Here's the drawing with two shaded views (mm, measured from the low corner). I have some questions. A direction names the side the tool comes from. Give positions to 0.01 mm unless a question says otherwise; leave off trailing zeros. Order: outer loops, then holes, each group sorted by start corner. A loop starts at its lowest first (then second) coordinate and runs counter-clockwise, first axis right, second up. Notation, with made-up numbers: (-32.75, 31) - (-7.75, 31) arc R21 cw to (-7.75, 37) - close; hole circle Ø10 at (61, 82.5). An arc over 180 degrees is marked (long way). Use one line per item in the form item = value. Start each with the question number.
1) For pin 1 (6.5 mm diameter, centred on y = 9.5, z = 13.5, fed in from +X); pin 2 (3 mm diameter, centred on x = 6.35, z = 6.35, fed in from -Y); pin 3 (4 mm diameter, centred on x = 22, y = 3.5, fed in from +Z), each with a flat end and sliding along its axis, tell me the tip position at first contact or that it passes through.
2) Suppose I cut it at A-A, the plane x = 6.35. Write out the boundary of the cut face in (y, z), and give its area (3 significant figures).
3) Please list where these lines run through material, in increasing order: probe 1 along Z at (x, y) = (6.35, 6.5); probe 2 along Z at (x, y) = (3.25, 6.35); probe 3 along Z at (x, y) = (6.35, 5).
4) Which directions (+Z, -Z, +X, -X, +Y, -Y) give clear straight access to the entire face, cutting with the end or side of a thin tool? Please do the marked faces 5 and 6.
5) We'd pull the mould along Y, two halves only. Please class the marked faces 1, 2, 3 and 4: released by +Y, released by -Y, zero draft, split by the parting line, or undercut.
6) Suppose I cut it at C-C, the plane z = 6.35. Write out the boundary of the cut face in (x, y), and give its area (3 significant figures).
7) Suppose I cut it at B-B, the plane y = 6.35. Write out the boundary of the cut face in (x, z), and give its area (3 significant figures).
8) Suppose I cut it at D-D, the plane x = 3. Write out the boundary of the cut face in (y, z), and give its area (3 significant figures).
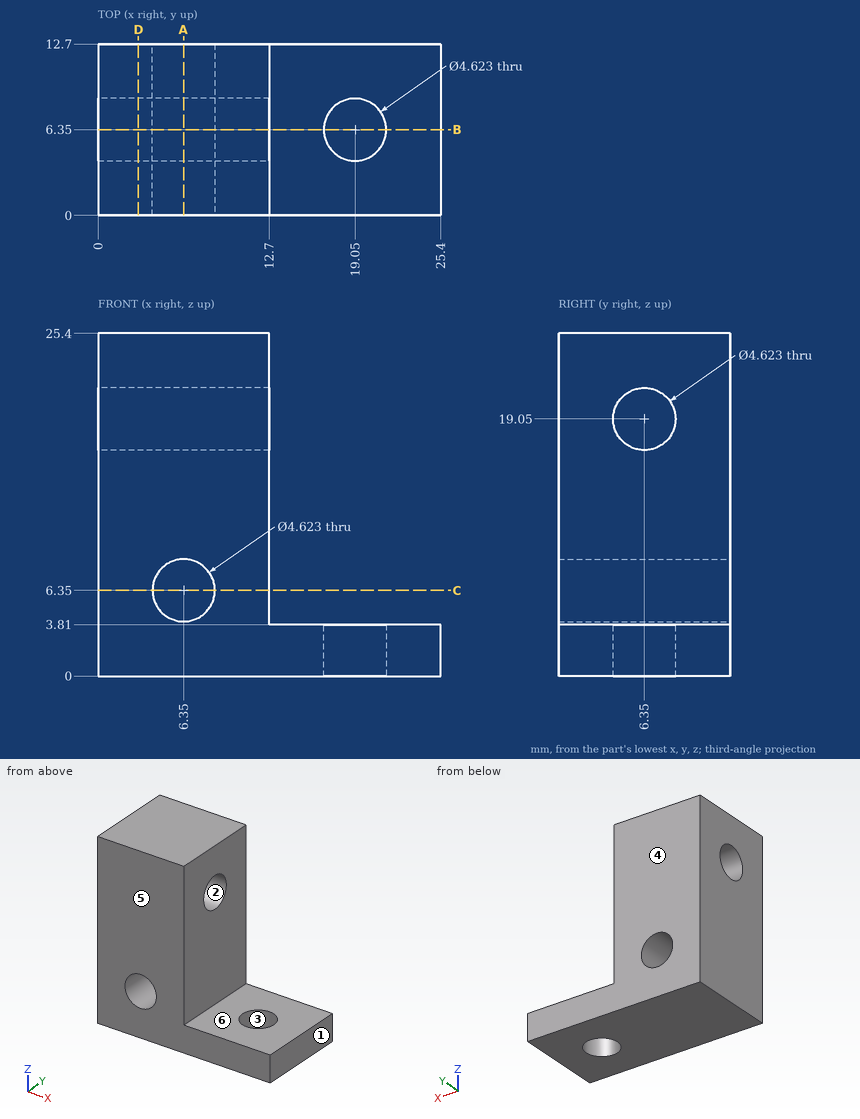
Result sheet:
q1.pin_1 = 12.7
q1.pin_2 = through
q1.pin_3 = 3.81
q2.outline = (0, 0) - (12.7, 0) - (12.7, 4.04) - (0, 4.04) - close; (0, 8.66) - (12.7, 8.66) - (12.7, 25.4) - (0, 25.4) - close; hole circle Ø4.62 at (6.35, 19.05)
q2.area = 247 mm²
q3.probe_1 = 0 to 4.04, 8.66 to 16.74, 21.36 to 25.4
q3.probe_2 = 0 to 16.74, 21.36 to 25.4
q3.probe_3 = 0 to 4.04, 8.66 to 17.17, 20.93 to 25.4
q4.face_5 = +Z, -Z, +X, -X, -Y
q4.face_6 = +Z, +X, +Y, -Y
q5.face_1 = zero draft
q5.face_2 = undercut
q5.face_3 = undercut
q5.face_4 = released by +Y
q6.outline = (0, 0) - (4.04, 0) - (4.04, 12.7) - (0, 12.7) - close; (8.66, 0) - (12.7, 0) - (12.7, 12.7) - (8.66, 12.7) - close
q6.area = 103 mm²
q7.outline = (0, 0) - (16.74, 0) - (16.74, 3.81) - (12.7, 3.81) - (12.7, 16.74) - (0, 16.74) - close; (0, 21.36) - (12.7, 21.36) - (12.7, 25.4) - (0, 25.4) - close; (21.36, 0) - (25.4, 0) - (25.4, 3.81) - (21.36, 3.81) - close; hole circle Ø4.62 at (6.35, 6.35)
q7.area = 278 mm²
q8.outline = (0, 0) - (12.7, 0) - (12.7, 25.4) - (0, 25.4) - close; hole circle Ø4.62 at (6.35, 19.05)
q8.area = 306 mm²
